For this review, take the finished solid that the model builds, in its own axes (mm). Give positions to 0.01 mm unless a question says otherwise; leave off trailing zeros. Write each loop counter-clockwise with the first axis right and the second up, starting at its lowest first coordinate (ties: lowest second). Pieces come first, ordered by that corner, then holes.
1) We need section B-B on z = 4. Give the boundary of the cut face in (x, y), and give its area (3 significant figures).
2) For P1, Ø7.5, axis at x = -63.5, y = 236.5, coming from the -Z side (3 decimals), flat-tipped, find the tip position at first contact; note if it passes through.
3) Wall thickness on line 1 along Y through (x, z) = (51, 9): over which ranges is the line inside the solid? List them lowest first.
4) We need section A-A on x = 0.5. Give the boundary of the cut face in (y, z) (3 decimals), and give its area (3 significant figures).
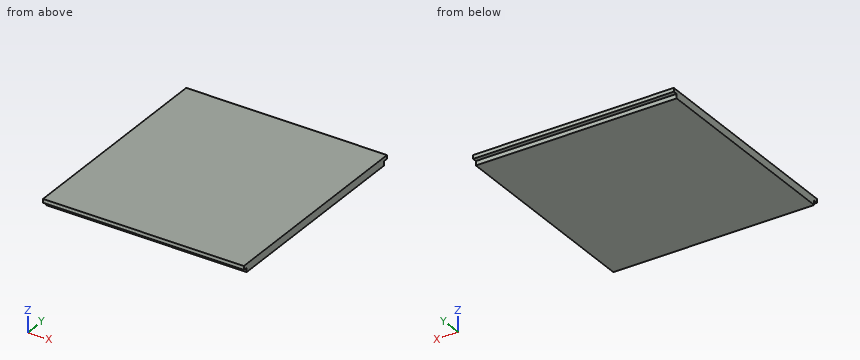
from build123d import *

# Parameters (mm, degrees)
F0_W     = 444.5
F0_H     = 482.6
F1_DEPTH = 17.78
F2_W     = 9.525
F2_H     = 9.525
F3_DEPTH = 444.5


# Not quite as in the source:
# - a feature of the source that left no trace in its solid (it failed there, or was rolled back) is left out


with BuildPart() as f1:
    # F0 (on Top) → F1 (new body)
    with BuildSketch(Plane.XY):
        with Locations((-25.2657681704, 0.1800126585)):
            Rectangle(F0_W, F0_H)
    extrude(amount=F1_DEPTH)

    # F2 (on face) → F3 (cut)
    with BuildSketch(Plane.YZ.offset(196.9842318296)):
        with Locations((236.7175126585, 4.7625)):
            Rectangle(F2_W, F2_H)
        with Locations((-236.3574873415, 4.7625)):
            Rectangle(F2_W, F2_H)
    extrude(amount=-F3_DEPTH, mode=Mode.SUBTRACT)


solid = f1.part
Results list:
1. outline: (-247.52, -231.59) - (196.98, -231.59) - (196.98, 231.96) - (-247.52, 231.96) - close
1. area: 206,000 mm2
2. P1: stops at z = 9.525
3. line 1: y = -231.59 to 231.96
4. outline: (-241.12, 9.525) - (-231.595, 9.525) - (-231.595, 0) - (231.955, 0) - (231.955, 9.525) - (241.48, 9.525) - (241.48, 17.78) - (-241.12, 17.78) - close
4. area: 8,400 mm2
